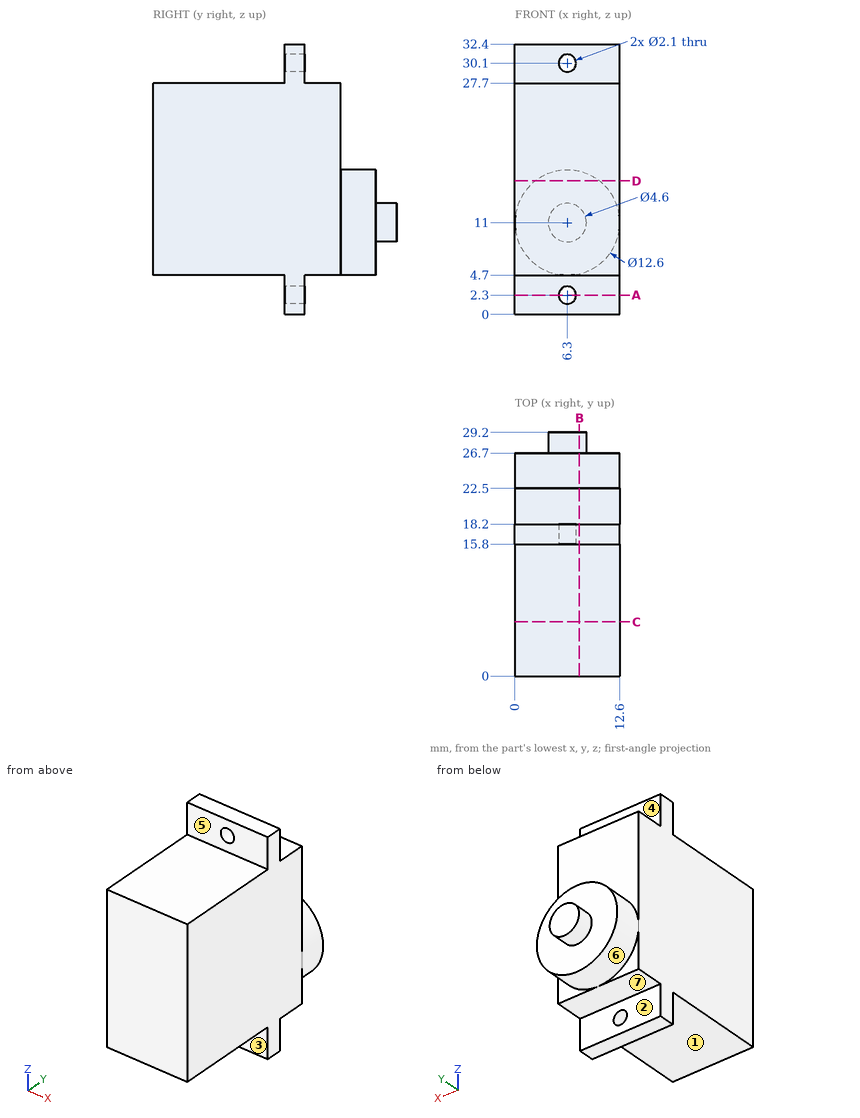
The drawing under review shows one solid part. Ordinate dimensions are in mm from its lowest x, y, z. A direction names the side the tool comes from. Coordinates: 2 decimals unless noted, no trailing zeros. Order: outer loops, then holes, each group sorted by start corner. A loop starts at its lowest first (then second) coordinate and runs counter-clockwise, first axis right, second up. Notation, with made-up numbers: (-26, 32) -> (10, 32) arc R17 cw to (10, 56) -> close; hole circle Ø10 at (80, 16.25). An arc over 180 degrees is marked (long way). Answer in a Markdown table with one row per item.
(1) Consider section B-B (x = 7.75). Write out the cut boundary in (y, z), plus the area to 3 significant figures.
Answers:
| item | result |
|---|---|
| outline | (0, 4.7) -> (15.8, 4.7) -> (15.8, 0) -> (18.2, 0) -> (18.2, 4.7) -> (22.5, 4.7) -> (22.5, 4.87) -> (26.7, 4.87) -> (26.7, 9.21) -> (29.2, 9.21) -> (29.2, 12.79) -> (26.7, 12.79) -> (26.7, 17.13) -> (22.5, 17.13) -> (22.5, 27.7) -> (18.2, 27.7) -> (18.2, 32.4) -> (15.8, 32.4) -> (15.8, 27.7) -> (0, 27.7) -> close |
| area | 600 mm² |
(2) Consider section D-D (z = 16). Write out the cut boundary in (x, y).
Answers:
| item | result |
|---|---|
| outline | (0, 0) -> (12.6, 0) -> (12.6, 22.5) -> (10.13, 22.5) -> (10.13, 26.7) -> (2.47, 26.7) -> (2.47, 22.5) -> (0, 22.5) -> close |
(3) The part is to be moulded in two halves that separate along Y. For the marked faces 1, 2 and 3, say which applies: +Y half, -Y half, draft (parallel to the pull), parting line (faces both ways), or undercut.
Answers:
| item | result |
|---|---|
| face 1 | draft |
| face 2 | +Y half |
| face 3 | -Y half |
(4) Machinability: for the marked faces 4, 5, 6 and 7, which of the approach directions +Z, -Z, +X, -X, +Y, -Y give a long, thin tool a straight path to every point of the face, cutting with its end or side? Answer none if there is none.
Answers:
| item | result |
|---|---|
| face 4 | +Z, +X, -X, +Y |
| face 5 | +Z, +X, -X, -Y |
| face 6 | +Y |
| face 7 | -Z, +X, -X, +Y |
(5) Insertion check: pin 1 (2 mm diameter, centred on x = 6.5, z = 16, fed in from +Y); pin 2 (2 mm diameter, centred on x = 5.5, y = 20, fed in from +Z); pin 3 (1.4 mm diameter, centred on x = 3.5, z = 1.5, fed in from +Y). Each pin has a flat end and moves straight along its axis. Give the tip position at first contact, or say it passes through.
Answers:
| item | result |
|---|---|
| pin 1 | y = 26.7 |
| pin 2 | z = 27.7 |
| pin 3 | y = 18.2 |
(6) Wall thickness on line 1 along Z through (x, y) = (6.3, 16.85); line 2 along Y through (x, z) = (5.75, 4.5); line 3 along Z through (x, y) = (5.5, 17): over which ranges is each line inside the solid? List them lowest first.
Answers:
| item | result |
|---|---|
| line 1 | 0 to 1.25, 3.35 to 29.05, 31.15 to 32.4 |
| line 2 | 15.8 to 18.2 |
| line 3 | 0 to 1.62, 2.98 to 29.42, 30.78 to 32.4 |
(7) Consider section C-C (y = 6.5). Write out the cut boundary in (x, z).
Answers:
| item | result |
|---|---|
| outline | (0, 4.7) -> (12.6, 4.7) -> (12.6, 27.7) -> (0, 27.7) -> close |
(8) Consider section A-A (z = 2.3). Write out the cut boundary in (x, y).
Answers:
| item | result |
|---|---|
| outline | (0, 15.8) -> (5.25, 15.8) -> (5.25, 18.2) -> (0, 18.2) -> close; (7.35, 15.8) -> (12.6, 15.8) -> (12.6, 18.2) -> (7.35, 18.2) -> close |
